Part model, mm, in its own coordinate system. Face numbers are marked on the shaded views. Coordinates: 2 decimals unless noted, no trailing zeros. Loops run counter-clockwise (first coordinate to the right, second up) from the corner with the lowest first, then second, coordinate; pieces in that order, holes last. Notation, with made-up numbers: (-31, -26) - (8, -26) arc R12 ccw to (8, -14) - close; hole circle Ø3 at (69.25, 16.25). An arc over 180 degrees is marked (long way). Answer as CSV lines item,"result".
from build123d import *

# Parameters (mm, degrees)
F0_W     = 200
F0_H     = 75
F1_DEPTH = 10
F2_W     = 10
F2_H     = 50
F3_DEPTH = 5
F4_W     = 35
F4_H     = 55
F4_W_2   = 9
F4_H_2   = 9
F5_DEPTH = 5


with BuildPart() as f1:
    # F0 (on Top) → F1 (new body)
    with BuildSketch(Plane.XY):
        Rectangle(F0_W, F0_H)
    extrude(amount=F1_DEPTH)

    # F2 (on face) → F3 (cut)
    with BuildSketch(Plane.XY.offset(10)):
        with Locations((-70, 0)):
            Rectangle(F2_W, F2_H)
        with Locations((27.5, 0)):
            Rectangle(F2_W, F2_H)
        with Locations((87.5, 0)):
            Rectangle(F2_W, F2_H)
    extrude(amount=-F3_DEPTH, mode=Mode.SUBTRACT)

    # F4 (on face) → F5 (cut)
    with BuildSketch(Plane.XY.offset(10)):
        with Locations((-20.039216, 0)):
            Rectangle(F4_W, F4_H)
        with Locations((14.87713, -33)):
            Rectangle(F4_W_2, F4_H_2)
    extrude(amount=-F5_DEPTH, mode=Mode.SUBTRACT)


solid = f1.part
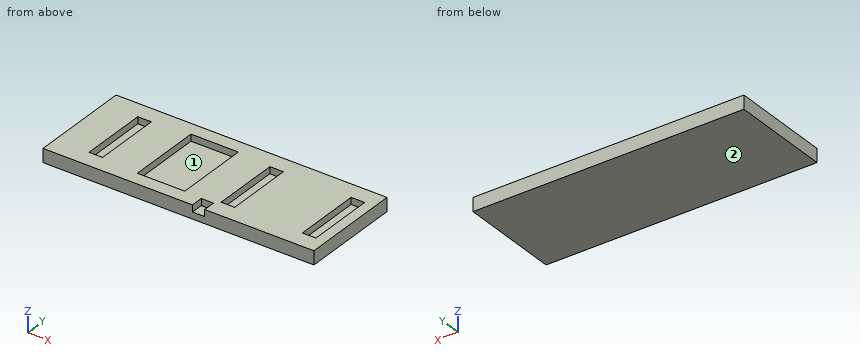
Q1. Saw through at D-D (x = 27). Give the cut face in (y, z).
Results:
outline,"(-37.5, 0) - (37.5, 0) - (37.5, 10) - (25, 10) - (25, 5) - (-25, 5) - (-25, 10) - (-37.5, 10) - close"
Q2. Saw through at C-C (y = -16). Give the cut face in (x, z).
Results:
outline,"(-100, 0) - (100, 0) - (100, 10) - (92.5, 10) - (92.5, 5) - (82.5, 5) - (82.5, 10) - (32.5, 10) - (32.5, 5) - (22.5, 5) - (22.5, 10) - (-2.54, 10) - (-2.54, 5) - (-37.54, 5) - (-37.54, 10) - (-65, 10) - (-65, 5) - (-75, 5) - (-75, 10) - (-100, 10) - close"
Q3. Saw through at A-A (z = 6.75). Give the cut face in (x, y).
Results:
outline,"(-100, -37.5) - (10.38, -37.5) - (10.38, -28.5) - (19.38, -28.5) - (19.38, -37.5) - (100, -37.5) - (100, 37.5) - (-100, 37.5) - close; hole (-75, -25) - (-65, -25) - (-65, 25) - (-75, 25) - close; hole (-37.54, -27.5) - (-2.54, -27.5) - (-2.54, 27.5) - (-37.54, 27.5) - close; hole (22.5, -25) - (32.5, -25) - (32.5, 25) - (22.5, 25) - close; hole (82.5, -25) - (92.5, -25) - (92.5, 25) - (82.5, 25) - close"
Q4. Wall check: L1, parallel to X at y = -17.5, z = 8.25; L2, parallel to Z at x = -24.5, y = 10; L3, parallel to Y at x = -36, z = 8.75. Give the ranges that are in metal, low to high.
Results:
L1,"x = -100 to -75, -65 to -37.54, -2.54 to 22.5, 32.5 to 82.5, 92.5 to 100"
L2,"z = 0 to 5"
L3,"y = -37.5 to -27.5, 27.5 to 37.5"
Q5. Flat gauge pins, fed straight in: pin 1 (1.5 mm diameter, centred on x = -72.5, y = 14.5, fed in from +Z); pin 2 (2.5 mm diameter, centred on x = 16.5, z = 6.5, fed in from -Y). Where does each tip first touch, or does it go through?
Results:
pin 1,"stops at z = 5"
pin 2,"stops at y = -28.5"
Q6. Two-plate mould, pull along Y, no slides. Class the marked faces 1 and 2: released by +Y, released by -Y, zero draft, split by the parting line, or undercut.
Results:
face 1,"undercut"
face 2,"zero draft"
Q7. Saw through at B-B (x = -19.5). Give the cut face in (y, z), then the cut area to 3 significant figures.
Results:
outline,"(-37.5, 0) - (37.5, 0) - (37.5, 10) - (27.5, 10) - (27.5, 5) - (-27.5, 5) - (-27.5, 10) - (-37.5, 10) - close"
area,"475 mm^2"
